from build123d import *

# Parameters (mm, degrees)
SKETCH1_R                       = 7.25
BOSS_EXTRUDE1_DEPTH             = 5
SKETCH2_R                       = 11.75
SKETCH2_R_2                     = 7.25
BOSS_EXTRUDE2_DEPTH             = 3.5
FILLET1_R                       = 4.5
FILLET2_R                       = 2.5
SKETCH3_R                       = 1.5
BOSS_EXTRUDE3_DEPTH             = 2.5
BOSS_EXTRUDE3_DIRECTION_2_REACH = 34
CBORE_FOR_M3_SBHCS1_D           = 3.4
CBORE_FOR_M3_SBHCS1_CBORE_D     = 6.7
CBORE_FOR_M3_SBHCS1_CBORE_DEPTH = 1.65
SKETCH6_R                       = 7.25
CUT_EXTRUDE1_DEPTH              = 3
SKETCH7_R                       = 9.5
CUT_EXTRUDE2_DEPTH              = 4.5
SKETCH10_R                      = 3
BOSS_EXTRUDE5_DEPTH             = 2
SKETCH11_R                      = 3
BOSS_EXTRUDE6_DEPTH             = 0.5
SKETCH12_R                      = 1.5
CUT_EXTRUDE4_DEPTH              = 4


with BuildPart() as part:
    # Sketch1 → Boss-Extrude1 (new body)
    with BuildSketch(Plane(origin=(0, 0, 0), x_dir=(0, 0, -1), z_dir=(1, 0, 0))):
        Polygon((-25, 16), (-25, 7.5), (-13.5, 7.5), (-13.5, -7.5), (-25, -7.5), (-25, -16), (25, -16), (25, 16), align=None)
        with Locations((7, 0)):
            Circle(SKETCH1_R, mode=Mode.SUBTRACT)
    extrude(amount=BOSS_EXTRUDE1_DEPTH)

    # Sketch2 → Boss-Extrude2 (add)
    with BuildSketch(Plane(origin=(5, 0, 0), x_dir=(0, 0, -1), z_dir=(1, 0, 0))):
        with Locations((7, 0)):
            Circle(SKETCH2_R)
        with Locations((7, 0)):
            Circle(SKETCH2_R_2, mode=Mode.SUBTRACT)
    extrude(amount=BOSS_EXTRUDE2_DEPTH)

    # Fillet1
    fillet1_edges = [part.edges().sort_by_distance(p)[0] for p in [
        (2.5, 16, 25),
        (2.5, 16, -25),
        (2.5, -16, -25),
        (2.5, -16, 25),
    ]]
    fillet(fillet1_edges, radius=FILLET1_R)

    # Fillet2
    fillet2_edges = [part.edges().sort_by_distance(p)[0] for p in [
        (2.5, 7.5, 13.5),
        (2.5, 7.5, 25),
        (2.5, -7.5, 25),
        (2.5, -7.5, 13.5),
    ]]
    fillet(fillet2_edges, radius=FILLET2_R)

    # Sketch3 → Boss-Extrude3 (add)
    with BuildSketch(Plane(origin=(0, -16, 0), x_dir=(-1, 0, 0), z_dir=(0, -1, 0))):
        with Locations((-2.5, -23)):
            Circle(SKETCH3_R)
        with Locations((-2.5, 23)):
            Circle(SKETCH3_R)
    extrude(amount=BOSS_EXTRUDE3_DEPTH)

    # Sketch3 → Boss-Extrude3 direction 2 (add, up to next)
    with BuildSketch(Plane(origin=(0, -16, 0), x_dir=(-1, 0, 0), z_dir=(0, -1, 0)), mode=Mode.PRIVATE) as boss_extrude3_direction_2_sk1:
        with Locations((-2.5, -23)):
            Circle(SKETCH3_R)
    boss_extrude3_direction_2_tool1 = extrude(boss_extrude3_direction_2_sk1.sketch, amount=-BOSS_EXTRUDE3_DIRECTION_2_REACH, mode=Mode.PRIVATE) - part.part
    add(boss_extrude3_direction_2_tool1.solids().sort_by_distance((2.5, -16, 23))[0])
    # Sketch3 → Boss-Extrude3 direction 2 (add, up to next)
    with BuildSketch(Plane(origin=(0, -16, 0), x_dir=(-1, 0, 0), z_dir=(0, -1, 0)), mode=Mode.PRIVATE) as boss_extrude3_direction_2_sk2:
        with Locations((-2.5, 23)):
            Circle(SKETCH3_R)
    boss_extrude3_direction_2_tool2 = extrude(boss_extrude3_direction_2_sk2.sketch, amount=-BOSS_EXTRUDE3_DIRECTION_2_REACH, mode=Mode.PRIVATE) - part.part
    add(boss_extrude3_direction_2_tool2.solids().sort_by_distance((2.5, -16, -23))[0])

    # CBORE for M3 SBHCS1 (through all)
    with Locations(Plane(origin=(5, 0, 0), x_dir=(0, 0, -1), z_dir=(1, 0, 0))):
        with Locations((-20.5, 11.5), (-20.5, -11.5), (20.5, 11.5), (20.5, -11.5)):
            CounterBoreHole(CBORE_FOR_M3_SBHCS1_D / 2, CBORE_FOR_M3_SBHCS1_CBORE_D / 2, CBORE_FOR_M3_SBHCS1_CBORE_DEPTH)

    # Sketch6 → Cut-Extrude1 (cut)
    with BuildSketch(Plane.ZY):
        with BuildLine():
            Line((11.5, 5), (11.5, 14))
            Line((11.5, 14), (-16.758342613, 14))
            ThreePointArc((-16.758342613, 14), (-16.19375696, 12.80624304), (-16, 11.5))
            ThreePointArc((-16, 11.5), (-18.378679656, 7.531373033), (-23, 7.758342613))
            Line((-23, 7.758342613), (-23, -7.758342613))
            ThreePointArc((-23, -7.758342613), (-18.378679656, -7.531373033), (-16, -11.5))
            ThreePointArc((-16, -11.5), (-16.19375696, -12.80624304), (-16.758342613, -14))
            Line((-16.758342613, -14), (11.5, -14))
            Line((11.5, -14), (11.5, -5))
            Line((11.5, -5), (11.5, 5))
        make_face()
        with Locations((-7, 0)):
            Circle(SKETCH6_R, mode=Mode.SUBTRACT)
    extrude(amount=-CUT_EXTRUDE1_DEPTH, mode=Mode.SUBTRACT)

    # Sketch7 → Cut-Extrude2 (cut)
    with BuildSketch(Plane.ZY.offset(-3)):
        with Locations((-7, 0)):
            Circle(SKETCH7_R)
    extrude(amount=-CUT_EXTRUDE2_DEPTH, mode=Mode.SUBTRACT)

    # Sketch10 → Boss-Extrude5 (add)
    with BuildSketch(Plane(origin=(5, 0, 0), x_dir=(0, 0, -1), z_dir=(1, 0, 0))):
        with Locations((-6.5, 0)):
            Circle(SKETCH10_R)
    extrude(amount=BOSS_EXTRUDE5_DEPTH)

    # Sketch11 → Boss-Extrude6 (add)
    with BuildSketch(Plane.ZY.offset(-3)):
        with Locations((6.5, 0)):
            Circle(SKETCH11_R)
    extrude(amount=BOSS_EXTRUDE6_DEPTH)

    # Sketch12 → Cut-Extrude4 (cut)
    with BuildSketch(Plane.ZY.offset(-2.5)):
        with Locations((6.5, 0)):
            Circle(SKETCH12_R)
    extrude(amount=-CUT_EXTRUDE4_DEPTH, mode=Mode.SUBTRACT)


solid = part.part
Could you check a few things on this model? Use its own coordinates, in mm. A direction names the side the tool comes from. Round coordinates to 2 decimals unless told otherwise and drop trailing zeros. Order: outer loops, then holes, each group sorted by start corner. A loop starts at its lowest first (then second) coordinate and runs counter-clockwise, first axis right, second up.
Q1. Imagine slicing it at A-A, the plane z = -7. List the corners of the cut face in (x, y) for me.
Geometry says:
outline: (0, -16) - (5, -16) - (5, -11.75) - (8.5, -11.75) - (8.5, -7.25) - (7.5, -7.25) - (7.5, -9.5) - (3, -9.5) - (3, -14) - (0, -14) - close; (0, 14) - (3, 14) - (3, 9.5) - (7.5, 9.5) - (7.5, 7.25) - (8.5, 7.25) - (8.5, 11.75) - (5, 11.75) - (5, 16) - (0, 16) - close
Q2. Which directions (+Z, -Z, +X, -X, +Y, -Y) give clear straight access to the entire face, cutting with the end or side of a thin tool? Please do faces 5 (the face through (6.5, 0, 6)), 6 (the face through (3.35, -13, -22)), 7 (the face through (3, -8, 24)), 8 (the face through (2.825, -16.614, 24.464)).
Geometry says:
face 5: -X
face 6: +X
face 7: +Z, +X, -X
face 8: -Y
Q3. I'm going to push flat-ended pins straight in: P1, Ø1.5, axis at y = 4.5, z = 5.5, coming from the +X side; P2, Ø2.5, axis at y = 0, z = 6.5, coming from the +X side; P3, Ø15, axis at y = 3.5, z = -4.5, coming from the -X side. Where does each tip first touch, or does it pass through?
Geometry says:
P1: stops at x = 5
P2: stops at x = 7
P3: stops at x = 3
Q4. Imagine slicing it at D-D, the plane x = 5.5. List the corners of the cut face in (y, z) for me.
Geometry says:
outline: (-2.26, 4.53) arc R11.75 ccw (long way) to (2.26, 4.53) arc R3 ccw (long way) to start; hole circle Ø19 at (0, -7); hole circle Ø3 at (0, 6.5)
Q5. Thinking about a two-plate mould opening in Y: for faces 1 (the face through (0, -1, 13)), 2 (the face through (2.535, 14.647, -23.717)), 3 (the face through (3, 6, 2)), 4 (the face through (2, 7.5, 19)), which applies, released by +Y, released by -Y, zero draft, split by the parting line, or undercut?
Geometry says:
face 1: zero draft
face 2: released by +Y
face 3: undercut
face 4: undercut
Q6. Please list where these lines run through material, in increasing order: probe 1 along Y at (x, z) = (4.45, -20.5); probe 2 along Y at (x, z) = (4.5, 20.5); probe 3 along Y at (x, z) = (1.65, 20.5).
Geometry says:
probe 1: y = -16 to -14.85, -8.15 to 8.15, 14.85 to 16
probe 2: y = -16 to -14.85, -8.15 to -7.5, 7.5 to 8.15, 14.85 to 16
probe 3: y = -16 to -13.2, -9.8 to -7.5, 7.5 to 9.8, 13.2 to 16
Q7. Imagine slicing it at C-C, the plane z = 6. List the corners of the cut face in (x, y) for me.
Geometry says:
outline: (0, -16) - (5, -16) - (5, -2.96) - (7, -2.96) - (7, 2.96) - (5, 2.96) - (5, 16) - (0, 16) - (0, 14) - (3, 14) - (3, 2.96) - (2.5, 2.96) - (2.5, 1.41) - (6.5, 1.41) - (6.5, -1.41) - (2.5, -1.41) - (2.5, -2.96) - (3, -2.96) - (3, -14) - (0, -14) - close
Q8. Imagine slicing it at B-B, the plane y = 5.5. List the corners of the cut face in (x, z) for me.
Geometry says:
outline: (0, -25) - (5, -25) - (5, -17.38) - (8.5, -17.38) - (8.5, -11.72) - (7.5, -11.72) - (7.5, -14.75) - (3, -14.75) - (3, -23) - (0, -23) - close; (0, 11.5) - (3, 11.5) - (3, 0.75) - (7.5, 0.75) - (7.5, -2.28) - (8.5, -2.28) - (8.5, 3.38) - (5, 3.38) - (5, 13.55) - (0, 13.55) - close
